```python
from build123d import *

# Parameters (mm, degrees)
SKETCH1_R               = 35.052
SKETCH1_R_2             = 22.352
BOSS_EXTRUDE2_DEPTH     = 12.7
CUT_EXTRUDE4_DEPTH      = 52.172017822
CUT_EXTRUDE4_DEPTH_BACK = 52.172017822
SKETCH4_W               = 50.006101534
SKETCH4_H               = 77.834708864
BOSS_EXTRUDE6_START     = -12.7
BOSS_EXTRUDE6_DEPTH     = 12.7
CUT_EXTRUDE5_DEPTH      = 93.599518977
CUT_EXTRUDE5_DEPTH_BACK = 93.599518977
SKETCH14_W              = 7.62
SKETCH14_H              = 7.62
CAVITY1_START           = 2.54
CAVITY1_DEPTH           = 2.54
CAVITY1_START_2         = 7.62
CAVITY1_2_DEPTH         = 2.54
SKETCH16_W              = 25.4
SKETCH16_H              = 12.7
BOSS_EXTRUDE8_DEPTH     = 7.62
CAVITY3_START           = -41.188715615
CAVITY3_OUTLINE_W       = 25.4
CAVITY3_OUTLINE_H       = 7.62
CAVITY3_DEPTH           = 2.54
CAVITY3_START_2         = -38.648715615
CAVITY3_2_OUTLINE_W     = 25.4
CAVITY3_2_OUTLINE_H     = 2.54
CAVITY3_2_DEPTH         = 2.54
CUT_EXTRUDE6_DEPTH      = 74.941076403
CUT_EXTRUDE6_DEPTH_BACK = 74.941076403


# Read off the part's stored shape, not the designer's step: Cavity1, Cavity3
with BuildPart() as part:
    # Sketch1 → Boss-Extrude2 (new body)
    with BuildSketch(Plane(origin=(0, 0, 0), x_dir=(1, 0, 0), z_dir=(0, 1, 0))):
        with Locations(Location((0, 0, 0), (0, 0, 270))):
            Circle(SKETCH1_R)
        with Locations(Location((0, 0, 0), (0, 0, 270))):
            Circle(SKETCH1_R_2, mode=Mode.SUBTRACT)
    extrude(amount=BOSS_EXTRUDE2_DEPTH)

    # Sketch4 → Cut-Extrude4 (cut, two sides: drawn at the far end of the back side and taken through both)
    with BuildSketch(Plane(origin=(0, 12.7, 0), x_dir=(1, 0, 0), z_dir=(0, 1, 0)).offset(-CUT_EXTRUDE4_DEPTH_BACK)):
        with Locations((24.88666989, 1.453038664)):
            Rectangle(SKETCH4_W, SKETCH4_H)
    extrude(amount=CUT_EXTRUDE4_DEPTH + CUT_EXTRUDE4_DEPTH_BACK, mode=Mode.SUBTRACT)

    # Sketch13 → Boss-Extrude6 (add)
    with BuildSketch(Plane(origin=(0, 12.7, 0), x_dir=(1, 0, 0), z_dir=(0, 1, 0)).offset(BOSS_EXTRUDE6_START)):
        with BuildLine():
            Line((-22.534267524, 26.848640397), (-22.534267524, 35.051806794))
            Line((-22.534267524, 35.051806794), (-59.151198439, 35.051806794))
            Line((-59.151198439, 35.051806794), (-59.151198439, -35.051806794))
            Line((-59.151198439, -35.051806794), (-22.534267524, -35.051806794))
            Line((-22.534267524, -35.051806794), (-22.534267524, -26.848640397))
            ThreePointArc((-22.534267524, -26.848640397), (-35.052, 0), (-22.534267524, 26.848640397))
        make_face()
        with BuildLine():
            ThreePointArc((-22.534267524, 26.848640397), (-12.045163053, 32.917423214), (-0.116380877, 35.051806794))
            Line((-0.116380877, 35.051806794), (-22.534267524, 35.051806794))
            Line((-22.534267524, 35.051806794), (-22.534267524, 26.848640397))
        make_face()
        with BuildLine():
            Line((-22.534267524, -35.051806794), (-0.116380877, -35.051806794))
            ThreePointArc((-0.116380877, -35.051806794), (-12.045163053, -32.917423214), (-22.534267524, -26.848640397))
            Line((-22.534267524, -26.848640397), (-22.534267524, -35.051806794))
        make_face()
    extrude(amount=BOSS_EXTRUDE6_DEPTH)

    # Sketch14 → Cut-Extrude5 (cut, two sides: drawn at the far end of the back side and taken through both)
    with BuildSketch(Plane.XY.offset(35.051806794).offset(-CUT_EXTRUDE5_DEPTH_BACK)):
        with Locations((-42.641198439, 6.35)):
            Rectangle(SKETCH14_W, SKETCH14_H)
    extrude(amount=CUT_EXTRUDE5_DEPTH + CUT_EXTRUDE5_DEPTH_BACK, mode=Mode.SUBTRACT)

    # Cavity1 outline → Cavity1 (cut)
    with BuildSketch(Plane(origin=(0, 0, 0), x_dir=(1, 0, 0), z_dir=(0, 1, 0)).offset(CAVITY1_START)):
        with BuildLine():
            Line((-2.656380877, 35.051806794), (-2.656380877, 22.289859607))
            Line((-2.656380877, 22.289859607), (-1.66555177, 22.289859607))
            ThreePointArc((-1.66555177, 22.289859607), (-0.891502639, 22.33421427), (-0.116380877, 22.351697016))
            Line((-0.116380877, 22.351697016), (-0.116380877, 35.051806794))
            Line((-0.116380877, 35.051806794), (-2.656380877, 35.051806794))
        make_face()
    extrude(amount=CAVITY1_DEPTH, mode=Mode.SUBTRACT)

    # Cavity1 2 outline → Cavity1 2 (cut)
    with BuildSketch(Plane(origin=(0, 0, 0), x_dir=(1, 0, 0), z_dir=(0, 1, 0)).offset(CAVITY1_START_2)):
        with BuildLine():
            Line((-2.656380877, 35.051806794), (-2.656380877, 22.289859607))
            Line((-2.656380877, 22.289859607), (-1.66555177, 22.289859607))
            ThreePointArc((-1.66555177, 22.289859607), (-0.891502639, 22.33421427), (-0.116380877, 22.351697016))
            Line((-0.116380877, 22.351697016), (-0.116380877, 35.051806794))
            Line((-0.116380877, 35.051806794), (-2.656380877, 35.051806794))
        make_face()
    extrude(amount=CAVITY1_2_DEPTH, mode=Mode.SUBTRACT)

    # Sketch16 → Boss-Extrude8 (add)
    with BuildSketch(Plane(origin=(0, 0, -35.051806794), x_dir=(-1, 0, 0), z_dir=(0, 0, -1))):
        with Locations((15.356380877, 6.35)):
            Rectangle(SKETCH16_W, SKETCH16_H)
    extrude(amount=BOSS_EXTRUDE8_DEPTH)

    # Cavity3 outline → Cavity3 (cut)
    with BuildSketch(Plane.XY.offset(CAVITY3_START)):
        with Locations((-15.356380877, 6.296394857)):
            Rectangle(CAVITY3_OUTLINE_W, CAVITY3_OUTLINE_H)
    extrude(amount=CAVITY3_DEPTH, mode=Mode.SUBTRACT)

    # Cavity3 2 outline → Cavity3 2 (cut)
    with BuildSketch(Plane.XY.offset(CAVITY3_START_2)):
        with Locations((-15.356380877, 6.296394857)):
            Rectangle(CAVITY3_2_OUTLINE_W, CAVITY3_2_OUTLINE_H)
    extrude(amount=CAVITY3_2_DEPTH, mode=Mode.SUBTRACT)

    # Sketch17 → Cut-Extrude6 (cut, two sides: drawn at the far end of the back side and taken through both)
    with BuildSketch(Plane(origin=(-0.116380877, 0, 0), x_dir=(0, 0, -1), z_dir=(1, 0, 0)).offset(-CUT_EXTRUDE6_DEPTH_BACK)):
        Polygon((-35.051806794, 8.979999947), (-31.955539721, 8.979999947), (-31.955539721, 12.349999947), (-30.365539721, 12.349999947), (-27.874781804, 8.734999947), (-27.874781804, 3.964999947), (-30.365539721, 0.349999947), (-31.955539721, 0.349999947), (-31.955539721, 3.719999947), (-35.051806794, 3.719999947), align=None)
    extrude(amount=CUT_EXTRUDE6_DEPTH + CUT_EXTRUDE6_DEPTH_BACK, mode=Mode.SUBTRACT)


solid = part.part
```
Part model, mm, in its own coordinate system. A direction names the side the tool comes from. Round coordinates to 2 decimals unless told otherwise and drop trailing zeros. Loops run counter-clockwise (first coordinate to the right, second up) from the corner with the lowest first, then second, coordinate; pieces in that order, holes last. Notation, with made-up numbers: (-17, 12) -> (0, 12) arc R32 cw to (0, 41) -> close; hole circle Ø11 at (25.5, 31). An arc over 180 degrees is marked (long way). Use a Markdown table: item, result.
1) Cut at C-C, the plane y = 6.5. List the corners of the cut face in (x, z).
The answers:
| item | result |
|---|---|
| outline | (-59.15, -35.05) -> (-46.45, -35.05) -> (-46.45, 27.87) -> (-59.15, 27.87) -> close; (-38.83, -35.05) -> (-28.06, -35.05) -> (-28.06, -36.11) -> (-2.66, -36.11) -> (-2.66, -35.05) -> (-0.12, -35.05) -> (-0.12, -22.35) arc R22.35 cw to (-0.12, 22.35) -> (-0.12, 27.87) -> (-38.83, 27.87) -> close; (-28.06, -42.67) -> (-2.66, -42.67) -> (-2.66, -41.19) -> (-28.06, -41.19) -> close |
2) Probe line 1 (X direction, y = 6, z = -28); line 2 (Z direction, x = -11, y = 11.5); line 3 (Z direction, x = -37.5, y = 8.5). List the from-to ranges inside material, lowest first. Write a range as [from, to].
The answers:
| item | result |
|---|---|
| line 1 | x = [-59.15, -46.45], [-38.83, -0.12] |
| line 2 | z = [-42.67, -19.46], [19.46, 29.78], [31.96, 35.05] |
| line 3 | z = [-35.05, 27.87] |
3) Cut at D-D, the plane x = -54.5. List the corners of the cut face in (y, z) (3 decimals).
The answers:
| item | result |
|---|---|
| outline | (0, -35.052) -> (12.7, -35.052) -> (12.7, 35.052) -> (8.98, 35.052) -> (8.98, 31.956) -> (12.35, 31.956) -> (12.35, 30.366) -> (8.735, 27.875) -> (3.965, 27.875) -> (0.35, 30.366) -> (0.35, 31.956) -> (3.72, 31.956) -> (3.72, 35.052) -> (0, 35.052) -> close |
4) Drop flat-ended pins along their axis: pin 1 Ø1.5 at (x, y) = (-30.5, 6) entering from +Z; pin 2 Ø1.7 at (x, y) = (-38.5, 2.5) entering from -Z. Give the stop position or say it passes through.
The answers:
| item | result |
|---|---|
| pin 1 | stops at z = 27.87 |
| pin 2 | stops at z = -35.05 |
5) Tool access for faces 1 (the flat face through (-30, 2, 31.956)), 2 (the flat face through (-1, 1, -35.052)), 3 (the flat face through (-47, 6, -35.052)), 4 (the flat face through (-1, 7.62, -29)), 5 (the flat face through (-53, 3.72, 33)): list every direction of +Z, -Z, +X, -X, +Y, -Y with a clear straight run to the whole face (end or side of a thin tool).
The answers:
| item | result |
|---|---|
| face 1 | +X, -X |
| face 2 | -Z, +X, +Y, -Y |
| face 3 | -Z, -X, +Y, -Y |
| face 4 | -Z, +X |
| face 5 | +Z, +X, -X |
6) Pull direction Z, two halves, no side cores. Call faces 6 (the flat face through (-53, 8.98, 34)), 7 (the flat face through (-16, 9, -38.649)), 8 (the flat face through (-1, 6, -35.052)): pulls with the +Z half, pulls with the -Z half, needs draft (parallel to the pull), parting line crosses it, or undercut.
The answers:
| item | result |
|---|---|
| face 6 | needs draft |
| face 7 | undercut |
| face 8 | pulls with the -Z half |
7) Cut at A-A, the plane x = -14. List the corners of the cut face in (y, z) (3 decimals).
The answers:
| item | result |
|---|---|
| outline | (0, -42.672) -> (12.7, -42.672) -> (12.7, -17.424) -> (0, -17.424) -> close; (0, 17.424) -> (12.7, 17.424) -> (12.7, 35.052) -> (8.98, 35.052) -> (8.98, 31.956) -> (12.35, 31.956) -> (12.35, 30.366) -> (8.735, 27.875) -> (3.965, 27.875) -> (0.35, 30.366) -> (0.35, 31.956) -> (3.72, 31.956) -> (3.72, 35.052) -> (0, 35.052) -> close; hole (2.486, -41.189) -> (10.106, -41.189) -> (10.106, -38.649) -> (7.566, -38.649) -> (7.566, -36.109) -> (5.026, -36.109) -> (5.026, -38.649) -> (2.486, -38.649) -> close |
8) Cut at B-B, the plane z = 0. List the corners of the cut face in (x, y).
The answers:
| item | result |
|---|---|
| outline | (-59.15, 0) -> (-22.35, 0) -> (-22.35, 12.7) -> (-59.15, 12.7) -> close; hole (-46.45, 2.54) -> (-38.83, 2.54) -> (-38.83, 10.16) -> (-46.45, 10.16) -> close |
